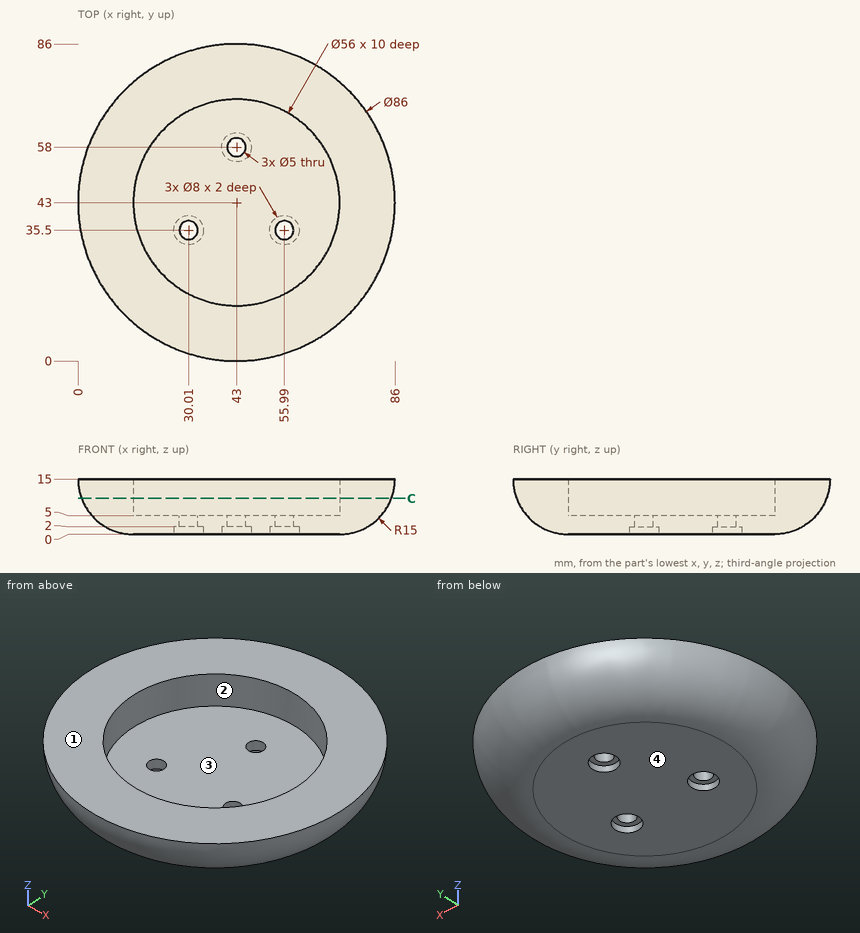
The drawing under review shows one solid part. Ordinate dimensions are in mm from its lowest x, y, z. A direction names the side the tool comes from. Coordinates: 2 decimals unless noted, no trailing zeros. Order: outer loops, then holes, each group sorted by start corner. A loop starts at its lowest first (then second) coordinate and runs counter-clockwise, first axis right, second up. Notation, with made-up numbers: (-33.75, 85) -> (8.25, 85) arc R11 cw to (8.25, 99) -> close; hole circle Ø3 at (46.25, -8). An arc over 180 degrees is marked (long way). Answer in a Markdown table with one row per item.
(1) Wall thickness on line 1 along Z through (x, y) = (33, 69.5); line 2 along Y through (x, z) = (22.5, 12) (1 decimal); line 3 along Z through (x, y) = (29.5, 66): over which ranges is each line inside the solid? List them lowest first.
Answers:
| item | result |
|---|---|
| line 1 | 0 to 15 |
| line 2 | 5.5 to 23.9, 62.1 to 80.5 |
| line 3 | 0 to 5 |
(2) Consider section C-C (z = 9.75). Write out the cut boundary in (x, y), plus the area to 3 significant figures.
Answers:
| item | result |
|---|---|
| outline | circle Ø84.1 at (43, 43); hole circle Ø56 at (43, 43) |
| area | 3,090 mm² |
(3) The part is to be moulded in two halves that separate along X. For the marked faces 3 and 4, say which applies: +X half, -X half, draft (parallel to the pull), parting line (faces both ways), or undercut.
Answers:
| item | result |
|---|---|
| face 3 | undercut |
| face 4 | draft |
(4) Machinability: for the marked faces 1 and 2, which of the approach directions +Z, -Z, +X, -X, +Y, -Y give a long, thin tool a straight path to every point of the face, cutting with its end or side? Answer none if there is none.
Answers:
| item | result |
|---|---|
| face 1 | +Z, +X, -X, +Y, -Y |
| face 2 | +Z |
(5) Insertion check: pin 1 (6 mm diameter, centred on y = 22, z = 5, fed in from +X); pin 2 (8 mm diameter, centred on x = 30.01, y = 35.5, fed in from +Z); pin 3 (3 mm diameter, centred on y = 66.5, z = 9.5, fed in from +X). Each pin has a flat end and moves straight along its axis. Give the tip position at first contact, or say it passes through.
Answers:
| item | result |
|---|---|
| pin 1 | x = 79.15 |
| pin 2 | z = 5 |
| pin 3 | x = 78.92 |
